The model under review builds one solid part; all positions refer to its coordinate system, in mm. A direction names the side the tool comes from. Coordinates: 2 decimals unless noted, no trailing zeros. Write each loop counter-clockwise with the first axis right and the second up, starting at its lowest first coordinate (ties: lowest second). Pieces come first, ordered by that corner, then holes. Notation, with made-up numbers: M 15,44 L 41,44 A3 cw 41,48 Z; hole C 37,13 d1. An arc over 180 degrees is marked long. Answer as a JSON object with one key per item and string values.
```python
from build123d import *

# Parameters (mm, degrees)
BOSS_EXTRUDE1_DEPTH                             = 6
FILLET1_R                                       = 3
CSK_FOR_M3_FLAT_HEAD_MACHINE_SCREW1_D           = 3.6
CSK_FOR_M3_FLAT_HEAD_MACHINE_SCREW1_CSINK_D     = 6.3
CSK_FOR_M3_FLAT_HEAD_MACHINE_SCREW1_CSINK_ANGLE = 90
SKETCH5_W                                       = 95
SKETCH5_H                                       = 95
BOSS_EXTRUDE2_DEPTH                             = 2
SKETCH6_R                                       = 2.25
BOSS_EXTRUDE3_DEPTH                             = 2
M3_CLEARANCE_HOLE1_D                            = 3.2
M3_CLEARANCE_HOLE1_DEPTH                        = 5
M3_CLEARANCE_HOLE1_TIP                          = 0.96137699


with BuildPart() as part:
    # Sketch1 → Boss-Extrude1 (new body)
    with BuildSketch(Plane(origin=(0, 0, 0), x_dir=(1, 0, 0), z_dir=(0, 1, 0))):
        with BuildLine():
            Line((5, 0), (100, 0))
            ThreePointArc((100, 0), (103.535533906, 1.464466094), (105, 5))
            Line((105, 5), (105, 100))
            ThreePointArc((105, 100), (103.535533906, 103.535533906), (100, 105))
            Line((100, 105), (5, 105))
            ThreePointArc((5, 105), (1.464466094, 103.535533906), (0, 100))
            Line((0, 100), (0, 5))
            ThreePointArc((0, 5), (1.464466094, 1.464466094), (5, 0))
        make_face()
    extrude(amount=BOSS_EXTRUDE1_DEPTH)

    # Fillet1
    fillet1_edges = [part.edges().sort_by_distance(p)[0] for p in [
        (52.5, 0, -105),
        (103.535533906, 0, -103.535533906),
        (105, 0, -52.5),
        (103.535533906, 0, -1.464466094),
        (52.5, 0, 0),
        (1.464466094, 0, -1.464466094),
        (0, 0, -52.5),
        (1.464466094, 0, -103.535533906),
    ]]
    fillet(fillet1_edges, radius=FILLET1_R)

    # CSK for M3 Flat Head Machine Screw1 (through all)
    with Locations(Plane(origin=(8.535533906, 0, -8.535533906), x_dir=(0, 0, -1), z_dir=(0, -1, 0))):
        with Locations((0, 0), (87.928932188, 0), (87.928932188, 87.928932188), (0, 87.928932188)):
            CounterSinkHole(CSK_FOR_M3_FLAT_HEAD_MACHINE_SCREW1_D / 2, CSK_FOR_M3_FLAT_HEAD_MACHINE_SCREW1_CSINK_D / 2, counter_sink_angle=CSK_FOR_M3_FLAT_HEAD_MACHINE_SCREW1_CSINK_ANGLE)

    # Sketch5 → Boss-Extrude2 (add)
    with BuildSketch(Plane(origin=(0, 6, 0), x_dir=(1, 0, 0), z_dir=(0, 1, 0))):
        with BuildLine():
            Line((5.585786438, 3.585786438), (99.414213562, 3.585786438))
            ThreePointArc((99.414213562, 3.585786438), (100.828427125, 4.171572875), (101.414213562, 5.585786438))
            Line((101.414213562, 5.585786438), (101.414213562, 99.414213562))
            ThreePointArc((101.414213562, 99.414213562), (100.828427125, 100.828427125), (99.414213562, 101.414213562))
            Line((99.414213562, 101.414213562), (5.585786438, 101.414213562))
            ThreePointArc((5.585786438, 101.414213562), (4.171572875, 100.828427125), (3.585786438, 99.414213562))
            Line((3.585786438, 99.414213562), (3.585786438, 5.585786438))
            ThreePointArc((3.585786438, 5.585786438), (4.171572875, 4.171572875), (5.585786438, 3.585786438))
        make_face()
        with Locations((52.5, 52.5)):
            Rectangle(SKETCH5_W, SKETCH5_H, mode=Mode.SUBTRACT)
    extrude(amount=BOSS_EXTRUDE2_DEPTH)

    # Sketch6 → Boss-Extrude3 (add)
    with BuildSketch(Plane(origin=(0, 6, 0), x_dir=(1, 0, 0), z_dir=(0, 1, 0))):
        with Locations(Location((8.535533906, 52.5, 0), (0, 0, 270))):
            Circle(SKETCH6_R)
        with Locations(Location((52.5, 8.535533906, 0), (0, 0, 270))):
            Circle(SKETCH6_R)
        with Locations(Location((96.464466094, 52.5, 0), (0, 0, 270))):
            Circle(SKETCH6_R)
        with Locations(Location((52.5, 96.464466094, 0), (0, 0, 270))):
            Circle(SKETCH6_R)
    extrude(amount=BOSS_EXTRUDE3_DEPTH)

    # M3 Clearance Hole1
    with Locations(Plane(origin=(8.535533906, 8, -52.5), x_dir=(0, 0, 1), z_dir=(0, 1, 0))):
        with Locations((0, 0), (43.983643016, 44.044146607), (0, 87.928932188), (-43.964466094, 43.964466094)):
            Hole(M3_CLEARANCE_HOLE1_D / 2, depth=M3_CLEARANCE_HOLE1_DEPTH)
            with Locations((0, 0, -(M3_CLEARANCE_HOLE1_DEPTH + M3_CLEARANCE_HOLE1_TIP / 2))):  # 118° drill point
                Cone(0, M3_CLEARANCE_HOLE1_D / 2, M3_CLEARANCE_HOLE1_TIP, mode=Mode.SUBTRACT)


solid = part.part
```
(1) Wall thickness on line 1 along Z through (x, y) = (52.5, 5.65); line 2 along X through (y, z) = (6.45, -52.5); line 3 along X through (y, z) = (6.5, -34): over which ranges is each line inside the solid? List them lowest first. Write a range as from..to.
Results list:
{"line 1": "-105..-98.06, -94.86..-10.11, -6.92..0", "line 2": "3.59..5, 6.29..6.94, 10.14..10.79, 94.21..94.86, 98.06..98.71, 100..101.41", "line 3": "3.59..5, 100..101.41"}
(2) For faces 1 (the face through (97.985, 6.986, -54.158)), 2 (the face through (105, 4, -52)), list the 3-axis set-ups (+Z, -Z, +X, -X, +Y, -Y) from which the entire face can be reached by the end or side of a thin tool; tool diameter is ignored.
Results list:
{"face 1": "+Y", "face 2": "+Z, -Z, +X, +Y, -Y"}
(3) Add section A-A on z = -85. Give the boundary of the cut face in (x, y), and give its area (3 significant figures).
Results list:
{"outline": "M 0,3 A3 ccw 3,0 L 102,0 A3 ccw 105,3 L 105,6 L 101.41,6 L 101.41,8 L 100,8 L 100,6 L 5,6 L 5,8 L 3.59,8 L 3.59,6 L 0,6 Z", "area": "632 mm²"}
(4) Add section B-B on x = 86.5. Give the boundary of the cut face in (y, z), and give its area (3 significant figures).
Results list:
{"outline": "M 0,-102 A3 ccw 3,-105 L 6,-105 L 6,-101.41 L 8,-101.41 L 8,-100 L 6,-100 L 6,-5 L 8,-5 L 8,-3.59 L 6,-3.59 L 6,0 L 3,0 A3 ccw 0,-3 Z", "area": "632 mm²"}
(5) Draft analysis for pull direction Z (two halves, no side actions). For faces 3 (the face through (95.369, 3.708, -97.893)), 4 (the face through (95, 8, -51.5)), 5 (the face through (104, 4, -103)), state which applies: released by +Z, released by -Z, zero draft, split by the parting line, or undercut.
Results list:
{"face 3": "undercut", "face 4": "zero draft", "face 5": "released by -Z"}
(6) For pin 1 Ø1 at (y, z) = (7, -33.5) entering from -X; pin 2 Ø4.5 at (x, z) = (96.46, -96.46) entering from +Y; pin 3 Ø1.6 at (y, z) = (7, -75) entering from +X; pin 4 Ø2.5 at (x, z) = (52.58, -8.52) entering from -Y, all flat-tipped, find the tip position at first contact; note any pin that passes through.
Results list:
{"pin 1": "x = 3.59", "pin 2": "y = 6", "pin 3": "x = 101.41", "pin 4": "y = 0"}
